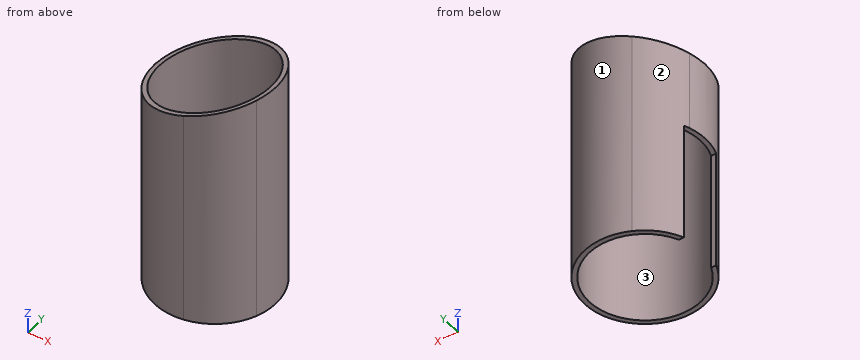
from build123d import *

# Parameters (mm, degrees)
F0_R          = 51.562
F0_R_2        = 47.5
F1_DEPTH      = 196.85
F3_DEPTH      = 61
F3_DEPTH_BACK = 74
F4_W          = 38.1
F4_H          = 101.6
F5_DEPTH      = 61
F7_DEPTH      = 222


with BuildPart() as f1:
    # F0 (on Top) → F1 (new body)
    with BuildSketch(Plane.XY):
        Circle(F0_R)
        Circle(F0_R_2, mode=Mode.SUBTRACT)
    extrude(amount=F1_DEPTH)

    # F2 (on Front) → F3 (cut, two sides)
    with BuildSketch(Plane.XZ) as f3_sk:
        Polygon((-53.913258, 197.321147), (-51.535871, 168.91), (53.578619, 197.321147), align=None)
    extrude(amount=F3_DEPTH, mode=Mode.SUBTRACT)
    extrude(f3_sk.sketch, amount=-F3_DEPTH_BACK, mode=Mode.SUBTRACT)

    # F4 (on Right) → F5 (cut)
    with BuildSketch(Plane.YZ):
        with Locations((0.965748, 50.8)):
            Rectangle(F4_W, F4_H)
    extrude(amount=-F5_DEPTH, mode=Mode.SUBTRACT)

    # F6 (on Top) → F7 (cut)
    with BuildSketch(Plane.XY):
        Polygon((-55.258796, 55.121914), (-55.258796, 0), (-55.258796, -56.109432), (54.045163, -56.109432), (54.045163, 51.900145), align=None)
        with BuildLine():
            ThreePointArc((-51.776279, 0), (-36.366122, 36.403048), (0, 51.900145))
            ThreePointArc((0, 51.900145), (36.452456, 36.489178), (51.776271, 0))
            ThreePointArc((51.776271, 0), (36.394792, -36.358057), (0, -51.652413))
            ThreePointArc((0, -51.652413), (-36.488721, -36.452209), (-51.776279, 0))
        make_face(mode=Mode.SUBTRACT)
    extrude(amount=F7_DEPTH, mode=Mode.SUBTRACT)


solid = f1.part
The listing builds one solid part. Answer for the finished solid, in the listing's coordinates (mm). Face numbers are marked on the shaded views. Round coordinates to 2 decimals unless told otherwise and drop trailing zeros. Loops run counter-clockwise (first coordinate to the right, second up) from the corner with the lowest first, then second, coordinate; pieces in that order, holes last. Notation, with made-up numbers: M 42,75.5 L 74,75.5 A9 cw 74,92.5 Z; hole C -5.75,17.5 d9. An arc over 180 degrees is marked long. Write each question's results on one line, items separated by ' | '. Start each with the question number.
1) Straight lines are drawn through the part: probe 1 along Y at (x, z) = (0, 129); probe 2 along Y at (x, z) = (-1, 51). For each, find the intervals that lie inside material, in ascending order.
2) Find section D-D on z = 113. Write down the section's boundary in (x, y).
3) Find section B-B on z = 23. Write down the section's boundary in (x, y), plus the area to 3 significant figures.
4) Each of these flat-tipped pins is pushed along its axis until it touches: pin 1 (2.5 mm diameter, centred on x = -48.5, y = 9.5, fed in from -Z); pin 2 (5 mm diameter, centred on x = -37.5, z = 49.5, fed in from +Y); pin 3 (2 mm diameter, centred on x = -45.5, z = 62.5, fed in from -Y). Where does it stop, or does it pass through?
5) Find section C-C on y = 38. Write down the section's boundary in (x, z), plus the area to 3 significant figures.
6) Find section A-A on x = -11. Write down the section's boundary in (y, z) (3 decimals).
7) Determine the mould class of the marked faces 1, 2 and 3 for opening direction X: pulls with the +X half, pulls with the -X half, needs draft (parallel to the pull), parting line crosses it, or undercut.
Final values:
1) probe 1: -51.56 to -47.5, 47.5 to 51.56 | probe 2: -51.55 to -47.49, 47.49 to 51.55
2) outline: M -49.16,15.56 A51.56 ccw 8.8,-50.81 A52.38 ccw 48.25,-18.18 A51.56 ccw -21.96,46.65 A52.79 ccw Z; hole C 0,0 d95
3) outline: M -48.29,-18.08 A51.56 ccw 8.8,-50.81 A52.38 ccw 48.25,-18.18 A51.56 ccw -21.96,46.65 A52.79 ccw -47.47,20.02 L -43.08,20.02 A47.5 cw long -43.92,-18.08 Z | area: 1,100 mm²
4) pin 1: z = 101.6 | pin 2: y = 37.72 | pin 3: y = -26.05
5) outline: M -34.7,0 L -28.5,0 L -28.5,175.14 L -34.7,173.46 Z; M 28.5,0 L 34.85,0 L 34.85,192.26 L 28.5,190.54 Z | area: 2,300 mm²
6) outline: M -50.375,0 L -46.209,0 L -46.209,179.866 L -50.375,179.866 Z; M 46.209,0 L 50.375,0 L 50.375,179.866 L 46.209,179.866 Z
7) face 1: parting line crosses it | face 2: pulls with the -X half | face 3: undercut
